For this review, use the dimensioned drawing (mm, ordinates from the lowest corner) and the shaded views. A direction names the side the tool comes from. Coordinates: 2 decimals unless noted, no trailing zeros. Write each loop counter-clockwise with the first axis right and the second up, starting at its lowest first coordinate (ties: lowest second). Pieces come first, ordered by that corner, then holes.
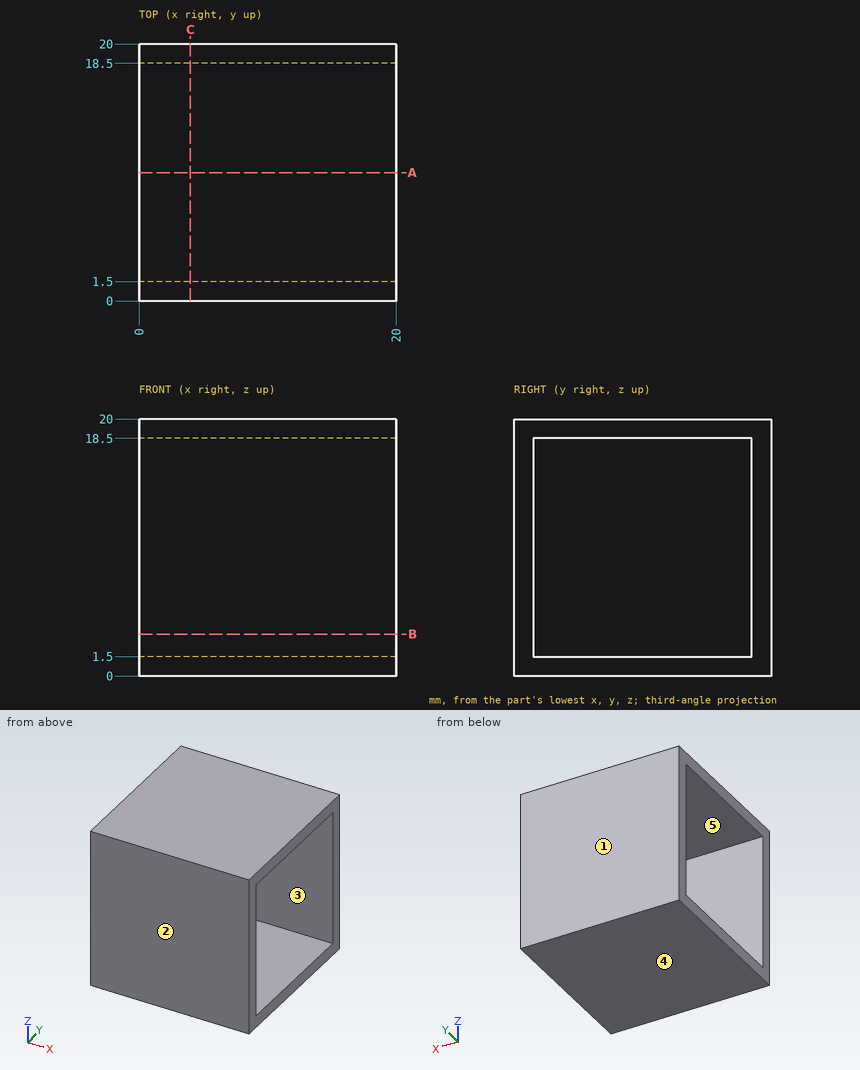
(1) Consider section C-C (x = 4). Give the boundary of the cut face in (y, z), plus the area to 3 significant figures.
(2) Mouldability with a two-part tool opening along Y and no side actions: class the marked faces 1, 2 and 3 as +Y half, -Y half, draft (parallel to the pull), parting line (faces both ways), or undercut.
(3) Wall thickness on line 1 (Y direction, x = 1.25, z = 2.25): over which ranges is the line inside the solid? List them lowest first.
(4) For the marked faces 4 and 5, list the 3-axis set-ups (+Z, -Z, +X, -X, +Y, -Y) from which the entire face can be reached by the end or side of a thin tool; tool diameter is ignored.
(5) Consider section A-A (y = 10). Give the boundary of the cut face in (x, z), plus the area to 3 significant figures.
Results:
1. outline: (0, 0) - (20, 0) - (20, 20) - (0, 20) - close; hole (1.5, 1.5) - (18.5, 1.5) - (18.5, 18.5) - (1.5, 18.5) - close
1. area: 111 mm2
2. face 1: +Y half
2. face 2: -Y half
2. face 3: undercut
3. line 1: y = 0 to 1.5, 18.5 to 20
4. face 4: -Z, +X, -X, +Y, -Y
4. face 5: +X, -X
5. outline: (0, 0) - (20, 0) - (20, 1.5) - (0, 1.5) - close; (0, 18.5) - (20, 18.5) - (20, 20) - (0, 20) - close
5. area: 60.0 mm2
